from build123d import *

# Parameters (mm, degrees)
BOSS_EXTRUDE1_DEPTH = 3.175
SKETCH2_R           = 2
CUT_EXTRUDE1_DEPTH  = 72.912172996
CUT_EXTRUDE2_START  = -3.175
CUT_EXTRUDE2_DEPTH  = 2
BOSS_EXTRUDE2_START = 10
BOSS_EXTRUDE2_DEPTH = 5
BOSS_EXTRUDE3_START = 30
BOSS_EXTRUDE3_DEPTH = 5


with BuildPart() as part:
    # Sketch1 → Boss-Extrude1 (new body)
    with BuildSketch(Plane(origin=(0, 0, 0), x_dir=(1, 0, 0), z_dir=(0, 1, 0))):
        Polygon((0, 0), (50.8, 0), (0, 50.8), align=None)
    extrude(amount=BOSS_EXTRUDE1_DEPTH)

    # Sketch2 → Cut-Extrude1 (cut, through all)
    with BuildSketch(Plane(origin=(0, 3.175, 0), x_dir=(1, 0, 0), z_dir=(0, 1, 0))):
        with Locations(Location((19.05, 6.35, 0), (0, 0, 270))):
            Circle(SKETCH2_R)
        with Locations(Location((6.35, 19.05, 0), (0, 0, 90))):
            Circle(SKETCH2_R)
    extrude(amount=-CUT_EXTRUDE1_DEPTH, mode=Mode.SUBTRACT)

    # Sketch3 → Cut-Extrude2 (cut)
    with BuildSketch(Plane(origin=(0, 3.175, 0), x_dir=(1, 0, 0), z_dir=(0, 1, 0)).offset(CUT_EXTRUDE2_START)):
        Polygon((8.370723055, 15.550005), (10.391446111, 19.05), (8.370723055, 22.549995), (4.329276945, 22.549995), (2.308553889, 19.05), (4.329276945, 15.550005), align=None)
        Polygon((22.549995, 4.329276945), (19.05, 2.308553889), (15.550005, 4.329276945), (15.550005, 8.370723055), (19.05, 10.391446111), (22.549995, 8.370723055), align=None)
    extrude(amount=CUT_EXTRUDE2_DEPTH, mode=Mode.SUBTRACT)

    # Sketch5 → Boss-Extrude2 (add)
    with BuildSketch(Plane(origin=(0, 0, 0), x_dir=(0, 0, -1), z_dir=(1, 0, 0)).offset(BOSS_EXTRUDE2_START)):
        Polygon((0, 0), (0, 3.175), (-50, 3.175), (-50, -2.5), (-75, -2.5), (-75, 3.175), (-80, 3.175), (-80, -5), (-47, -5), (-47, 0), align=None)
    extrude(amount=BOSS_EXTRUDE2_DEPTH)

    # Sketch5<3> → Boss-Extrude3 (add)
    with BuildSketch(Plane(origin=(0, 0, 0), x_dir=(0, 0, -1), z_dir=(1, 0, 0)).offset(BOSS_EXTRUDE3_START)):
        Polygon((0, 0), (0, 3.175), (-50, 3.175), (-50, -2.5), (-75, -2.5), (-75, 3.175), (-80, 3.175), (-80, -5), (-47, -5), (-47, 0), align=None)
    extrude(amount=BOSS_EXTRUDE3_DEPTH)


solid = part.part
Could you check a few things on this model? Use its own coordinates, in mm. A direction names the side the tool comes from. Give positions to 0.01 mm unless a question says otherwise; leave off trailing zeros. Order: outer loops, then holes, each group sorted by start corner. A loop starts at its lowest first (then second) coordinate and runs counter-clockwise, first axis right, second up.
Item 1: If we section it at A-A, the plane x = 6.35: Write out the boundary of the cut face in (y, z) (3 decimals).
Item 2: If we section it at C-C, the plane z = 31.5: Write out the boundary of the cut face in (x, y) (3 decimals), plus the area to 4 significant figures.
Item 3: If we section it at D-D, the plane x = 37.5: Write out the boundary of the cut face in (y, z) (3 decimals).
Item 4: I'm going to push flat-ended pins straight in: pin 1 (2 mm diameter, centred on y = 1, z = -6, fed in from +X); pin 2 (5.5 mm diameter, centred on x = 33.5, z = 62.5, fed in from +Y); pin 3 (1.5 mm diameter, centred on x = 43.5, y = -0.5, fed in from +Z). Where does each tip first touch, or does it pass through?
Item 5: If we mould it in two halves opening along Z, with no side actions, what happens to faces 6 (the face through (0, 2, -26)), 7 (the face through (6.262, 2.596, -17.052)), 8 (the face through (25.8, 1.6, -25)), 9 (the face through (21, 2, -5))? For each: pulls with the +Z half, pulls with the -Z half, needs draft (parallel to the pull), parting line crosses it, or undercut.
Item 6: If we section it at B-B, the plane z = 60: Write out the boundary of the cut face in (x, y).
Item 7: For faces 1 (the face through (22, 2, 0)), 2 (the face through (32, -2.5, 62)), 3 (the face through (43, 2, 0)), 4 (the face through (12, 3.175, 77)), 5 (the face through (14, 0, -3)), which set-ups out of +Z, -Z, +X, -X, +Y, -Y let a thin tool reach every point of the face, with its end or its side?
Item 8: I need wall thicknesses on line 1 (Y direction, x = 34, z = -3) (3 decimals); line 2 (Z direction, x = 6.35, y = 2.5); line 3 (Z direction, x = 19.5, y = 2.5). Which ranges of each line are inside material? Lowest first, please.
Values:
1. outline: (0, -44.45) - (3.175, -44.45) - (3.175, -21.05) - (2, -21.05) - (2, -22.55) - (0, -22.55) - close; (0, -15.55) - (2, -15.55) - (2, -17.05) - (3.175, -17.05) - (3.175, 0) - (0, 0) - close
2. outline: (10, 0) - (15, 0) - (15, 3.175) - (10, 3.175) - close; (30, 0) - (35, 0) - (35, 3.175) - (30, 3.175) - close
2. area: 31.75 mm2
3. outline: (0, -13.3) - (3.175, -13.3) - (3.175, 0) - (0, 0) - close
4. pin 1: stops at x = 45.8
4. pin 2: stops at y = -2.5
4. pin 3: stops at z = 0
5. face 6: needs draft
5. face 7: undercut
5. face 8: pulls with the -Z half
5. face 9: undercut
6. outline: (10, -5) - (15, -5) - (15, -2.5) - (10, -2.5) - close; (30, -5) - (35, -5) - (35, -2.5) - (30, -2.5) - close
7. face 1: +Z, +Y, -Y
7. face 2: +X, -X, +Y
7. face 3: +Z, +X, +Y, -Y
7. face 4: +Z, -Z, +X, -X, +Y
7. face 5: -Z, +X, -X, -Y
8. line 1: y = 0 to 3.175
8. line 2: z = -44.45 to -21.05, -17.05 to 0
8. line 3: z = -31.3 to -8.3, -4.4 to 0
